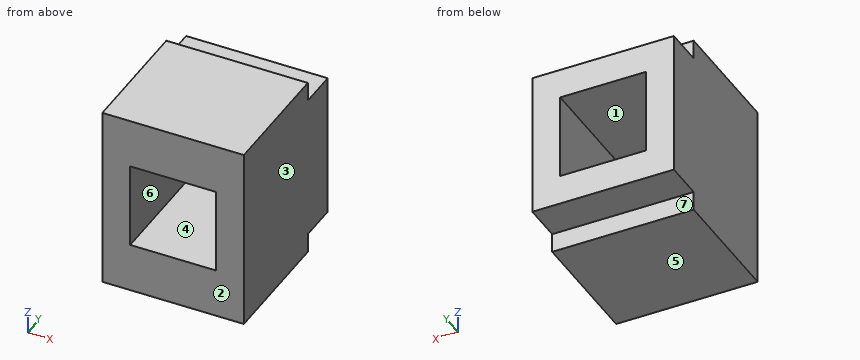
from build123d import *

# Parameters (mm, degrees)
SALIENTE_EXTRUIR1_DEPTH = 33
CROQUIS2_W              = 40
CROQUIS2_H              = 40
CORTAR_EXTRUIR1_DEPTH   = 94.348808241


with BuildPart() as part:
    # Croquis1 → Saliente-Extruir1 (new, symmetric)
    with BuildSketch(Plane(origin=(0, 0, 0), x_dir=(0, 0, -1), z_dir=(1, 0, 0))):
        Polygon((34, 38), (-34, 38), (-34, 20), (-43, 20), (-43, -38), (43, -38), (43, 20), (34, 20), align=None)
    extrude(amount=SALIENTE_EXTRUIR1_DEPTH, both=True)

    # Croquis2 → Cortar-Extruir1 (cut, through all)
    with BuildSketch(Plane(origin=(0, 38, 0), x_dir=(1, 0, 0), z_dir=(0, 1, 0))):
        Rectangle(CROQUIS2_W, CROQUIS2_H)
    extrude(amount=-CORTAR_EXTRUIR1_DEPTH, mode=Mode.SUBTRACT)


solid = part.part
Could you check a few things on this model? Use its own coordinates, in mm. Face numbers are marked on the shaded views. A direction names the side the tool comes from. Give positions to 0.01 mm unless a question says otherwise; leave off trailing zeros. Order: outer loops, then holes, each group sorted by start corner. A loop starts at its lowest first (then second) coordinate and runs counter-clockwise, first axis right, second up.
1. Suppose I cut it at B-B (x = 18.5). List the corners of the cut face in (y, z) for me.
2. Will these pins go through, and if not, where does the flat tip stop? P1, Ø9, axis at x = 3.5, y = 28.5, coming from the -Z side; P2, Ø9, axis at x = -5, y = 26, coming from the +Z side; P3, Ø7, axis at x = -2.5, z = 40, coming from the +Y side.
3. Suppose I cut it at C-C (y = 32). List the corners of the cut face in (x, z) for me, plus the area to 3 significant figures.
4. We'd pull the mould along X, two halves only. Please class the marked faces 1, 2, 3 and 4: pulls with the +X half, pulls with the -X half, needs draft (parallel to the pull), parting line crosses it, or undercut.
5. Suppose I cut it at A-A (z = -9). List the corners of the cut face in (x, y) for me.
6. I need wall thicknesses on L1, parallel to Z at x = -10, y = -23; L2, parallel to X at y = 13, z = 9.5; L3, parallel to Z at x = -4, y = 24. Which ranges of each line are inside material? Lowest first, please.
7. For the marked faces 5, 6 and 7, which set-ups out of +Z, -Z, +X, -X, +Y, -Y let a thin tool reach every point of the face, with its end or its side?
8. Suppose I cut it at D-D (x = -27). List the corners of the cut face in (y, z) for me, plus the area to 3 significant figures.
Solved:
1. outline: (-38, -43) - (20, -43) - (20, -34) - (38, -34) - (38, -20) - (-38, -20) - close; (-38, 20) - (38, 20) - (38, 34) - (20, 34) - (20, 43) - (-38, 43) - close
2. P1: stops at z = -34
2. P2: stops at z = 34
2. P3: stops at y = 20
3. outline: (-33, -34) - (33, -34) - (33, 34) - (-33, 34) - close; hole (-20, -20) - (20, -20) - (20, 20) - (-20, 20) - close
3. area: 2,890 mm2
4. face 1: undercut
4. face 2: needs draft
4. face 3: pulls with the +X half
4. face 4: undercut
5. outline: (-33, -38) - (-20, -38) - (-20, 38) - (-33, 38) - close; (20, -38) - (33, -38) - (33, 38) - (20, 38) - close
6. L1: z = -43 to -20, 20 to 43
6. L2: x = -33 to -20, 20 to 33
6. L3: z = -34 to -20, 20 to 34
7. face 5: -Z, +X, -X, +Y, -Y
7. face 6: +Y, -Y
7. face 7: -Z, +X, -X, +Y
8. outline: (-38, -43) - (20, -43) - (20, -34) - (38, -34) - (38, 34) - (20, 34) - (20, 43) - (-38, 43) - close
8. area: 6,210 mm2
